CAD build for the part. Positions are in the model's coordinates, mm. Give positions to 0.01 mm unless a question says otherwise; leave off trailing zeros. Order: outer loops, then holes, each group sorted by start corner. A loop starts at its lowest first (then second) coordinate and runs counter-clockwise, first axis right, second up. Notation, with made-up numbers: M -13,7.5 L 9,7.5 A22 cw 9,39.5 Z; hole C 20,19.5 d11. An arc over 180 degrees is marked long. Put each result on its own line as item: value. Start each with the question number.
1) Drill centre lines: line 1 (X direction, y = 1.7, z = -137.5); line 2 (Z direction, x = 113, y = 2) (3 decimals); line 3 (X direction, y = 0.35, z = -181.5). Where is each one in solid material? Low to high. Write a range as [from, to].
2) Cut at A-A (z = -129.5). Write the cut outline in (x, y) (3 decimals), and give its area (3 significant figures).
3) Pin check, flat tip, straight feed: pin 1 (1.6 mm diameter, centred on x = 313.5, y = 1, fed in from +Z). Stop position of the tip, or through.
4) Cut at D-D (y = 2.65). Give the number of separate pieces and of enclosed holes in the cut face, and give its area (3 significant figures).
5) Two-plate mould, pull along X, no slides. Class faces 1 (the face through (2.85, 1.61, -236.99)), 2 (the face through (207, 3.175, -122)), 3 (the face through (397.287, 1.565, -177.714)): released by +X, released by -X, zero draft, split by the parting line, or undercut.
6) Cut at C-C (x = 394). Write the cut outline in (y, z) (3 decimals).
7) Cut at B-B (x = 166.5). Write the cut outline in (y, z) (3 decimals).
```python
from build123d import *

# Parameters (mm, degrees)
SKETCH1_W           = 420
SKETCH1_H           = 240
SKETCH1_R           = 2.316650795
SKETCH1_R_2         = 5.401558945
SKETCH1_R_3         = 12
SKETCH1_R_4         = 1.8
SKETCH1_W_2         = 56.5
SKETCH1_H_2         = 56.5
SKETCH1_W_3         = 28
SKETCH1_H_3         = 28
BOSS_EXTRUDE1_DEPTH = 3.175
CUT_EXTRUDE1_DEPTH  = 10
FILLET1_R           = 10
SKETCH5_R           = 1.83
SKETCH5_R_2         = 2
SKETCH5_R_3         = 1.66
CUT_EXTRUDE2_DEPTH  = 3.175
SKETCH6_W           = 50
SKETCH6_H           = 3.175
CUT_EXTRUDE3_DEPTH  = 3.175


with BuildPart() as part:
    # Sketch1 → Boss-Extrude1 (new body)
    with BuildSketch(Plane(origin=(0, 0, 0), x_dir=(1, 0, 0), z_dir=(0, 1, 0))):
        with Locations((210, 120)):
            Rectangle(SKETCH1_W, SKETCH1_H)
        with Locations(Location((41, 182, 0), (0, 0, 270))):
            Circle(SKETCH1_R, mode=Mode.SUBTRACT)
        with Locations(Location((18.5, 169.009618943, 0), (0, 0, 270))):
            Circle(SKETCH1_R, mode=Mode.SUBTRACT)
        with Locations(Location((18.5, 194.990381057, 0), (0, 0, 270))):
            Circle(SKETCH1_R, mode=Mode.SUBTRACT)
        with Locations(Location((26, 182, 0), (0, 0, 270))):
            Circle(SKETCH1_R_2, mode=Mode.SUBTRACT)
        with Locations(Location((132, 37.5, 0), (0, 0, 270))):
            Circle(SKETCH1_R_3, mode=Mode.SUBTRACT)
        with Locations(Location((113, 37.5, 0), (0, 0, 270))):
            Circle(SKETCH1_R_4, mode=Mode.SUBTRACT)
        with Locations(Location((151, 37.5, 0), (0, 0, 270))):
            Circle(SKETCH1_R_4, mode=Mode.SUBTRACT)
        with Locations(Location((401.5, 194.990381057, 0), (0, 0, 90))):
            Circle(SKETCH1_R, mode=Mode.SUBTRACT)
        with Locations(Location((379, 182, 0), (0, 0, 90))):
            Circle(SKETCH1_R, mode=Mode.SUBTRACT)
        with Locations(Location((394, 182, 0), (0, 0, 90))):
            Circle(SKETCH1_R_2, mode=Mode.SUBTRACT)
        with Locations(Location((401.5, 169.009618943, 0), (0, 0, 90))):
            Circle(SKETCH1_R, mode=Mode.SUBTRACT)
        with Locations(Location((307, 37.5, 0), (0, 0, 90))):
            Circle(SKETCH1_R_4, mode=Mode.SUBTRACT)
        with Locations(Location((269, 37.5, 0), (0, 0, 90))):
            Circle(SKETCH1_R_4, mode=Mode.SUBTRACT)
        with Locations(Location((288, 37.5, 0), (0, 0, 90))):
            Circle(SKETCH1_R_3, mode=Mode.SUBTRACT)
        with Locations((171, 115)):
            Rectangle(SKETCH1_W_2, SKETCH1_H_2, mode=Mode.SUBTRACT)
        with Locations((93, 115)):
            Rectangle(SKETCH1_W_2, SKETCH1_H_2, mode=Mode.SUBTRACT)
        with Locations((327, 115)):
            Rectangle(SKETCH1_W_2, SKETCH1_H_2, mode=Mode.SUBTRACT)
        with Locations((249, 115)):
            Rectangle(SKETCH1_W_2, SKETCH1_H_2, mode=Mode.SUBTRACT)
        with Locations((210, 198)):
            Rectangle(SKETCH1_W_3, SKETCH1_H_3, mode=Mode.SUBTRACT)
    extrude(amount=BOSS_EXTRUDE1_DEPTH)

    # Sketch2 → Cut-Extrude1 (cut)
    with BuildSketch(Plane(origin=(0, 3.175, 0), x_dir=(1, 0, 0), z_dir=(0, 1, 0))):
        Polygon((0, 60), (0, 0), (80, 0), align=None)
        Polygon((420, 60), (420, 0), (340, 0), align=None)
    extrude(amount=-CUT_EXTRUDE1_DEPTH, mode=Mode.SUBTRACT)

    # Fillet1
    fillet1_edges = [part.edges().sort_by_distance(p)[0] for p in [
        (420, 1.5875, -60),
        (80, 1.5875, 0),
        (0, 1.5875, -60),
        (340, 1.5875, 0),
        (0, 1.5875, -240),
        (420, 1.5875, -240),
    ]]
    fillet(fillet1_edges, radius=FILLET1_R)

    # Sketch5 → Cut-Extrude2 (cut)
    with BuildSketch(Plane(origin=(0, 3.175, 0), x_dir=(1, 0, 0), z_dir=(0, 1, 0))):
        with Locations(Location((11, 229, 0), (0, 0, 270))):
            Circle(SKETCH5_R)
        with Locations(Location((11, 65.5, 0), (0, 0, 270))):
            Circle(SKETCH5_R_2)
        with Locations(Location((83.666666667, 11, 0), (0, 0, 270))):
            Circle(SKETCH5_R_2)
        with Locations(Location((409, 65.5, 0), (0, 0, 90))):
            Circle(SKETCH5_R_2)
        with Locations(Location((336.333333333, 11, 0), (0, 0, 90))):
            Circle(SKETCH5_R_2)
        with Locations(Location((210, 115, 0), (0, 0, 270))):
            Circle(SKETCH5_R_3)
        with Locations(Location((132, 115, 0), (0, 0, 270))):
            Circle(SKETCH5_R_3)
        with Locations(Location((288, 115, 0), (0, 0, 270))):
            Circle(SKETCH5_R_3)
        with Locations(Location((40, 222.825, 0), (0, 0, 270))):
            Circle(SKETCH5_R)
        with Locations(Location((380, 222.825, 0), (0, 0, 90))):
            Circle(SKETCH5_R)
        with Locations(Location((409, 229, 0), (0, 0, 90))):
            Circle(SKETCH5_R)
    extrude(amount=-CUT_EXTRUDE2_DEPTH, mode=Mode.SUBTRACT)

    # Sketch6 → Cut-Extrude3 (cut)
    with BuildSketch(Plane(origin=(0, 3.175, 0), x_dir=(1, 0, 0), z_dir=(0, 1, 0))):
        with Locations((125, 230.4125)):
            Rectangle(SKETCH6_W, SKETCH6_H)
        with Locations((295, 230.4125)):
            Rectangle(SKETCH6_W, SKETCH6_H)
    extrude(amount=-CUT_EXTRUDE3_DEPTH, mode=Mode.SUBTRACT)


solid = part.part
```
Solution:
1. line 1: [0, 64.75], [121.25, 142.75], [199.25, 220.75], [277.25, 298.75], [355.25, 420]
1. line 2: [-240, -232], [-228.825, -143.25], [-86.75, -39.3], [-35.7, 0]
1. line 3: [0, 20.62], [31.38, 38.74], [43.26, 376.74], [381.26, 388.62], [399.38, 420]
2. outline: M 0,0 L 64.75,0 L 64.75,3.175 L 0,3.175 Z; M 121.25,0 L 142.75,0 L 142.75,3.175 L 121.25,3.175 Z; M 199.25,0 L 220.75,0 L 220.75,3.175 L 199.25,3.175 Z; M 277.25,0 L 298.75,0 L 298.75,3.175 L 277.25,3.175 Z; M 355.25,0 L 420,0 L 420,3.175 L 355.25,3.175 Z
2. area: 616 mm²
3. pin 1: z = 0
4. separate pieces: 1
4. enclosed holes: 32
4. area: 80,700 mm²
5. face 1: released by -X
5. face 2: zero draft
5. face 3: undercut
6. outline: M 0,-240 L 3.175,-240 L 3.175,-187.402 L 0,-187.402 Z; M 0,-176.598 L 3.175,-176.598 L 3.175,-40.5 L 0,-40.5 Z
7. outline: M 0,-240 L 3.175,-240 L 3.175,-143.25 L 0,-143.25 Z; M 0,-86.75 L 3.175,-86.75 L 3.175,0 L 0,0 Z
